Source: CAD feature listing. Evaluate the final solid. Frame: model axes, mm. Face numbers are marked on the shaded views. Round coordinates to 2 decimals unless told otherwise and drop trailing zeros. Write each loop counter-clockwise with the first axis right and the second up, starting at its lowest first coordinate (ties: lowest second). Pieces come first, ordered by that corner, then holes.
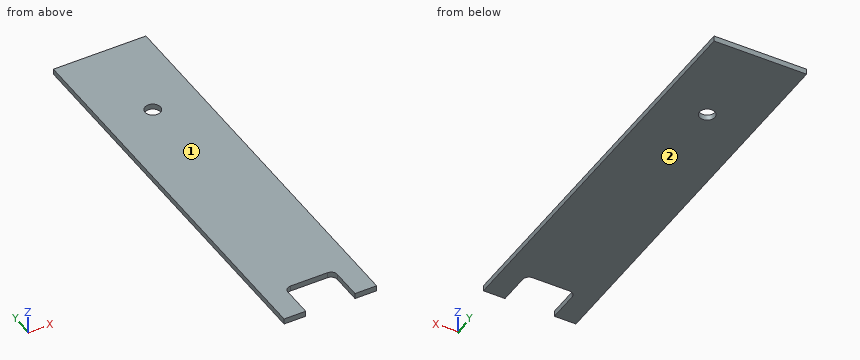
```python
from build123d import *

# Parameters (mm, degrees)
ESBO_O1_W                = 30
ESBO_O1_H                = 130
RESSALTO_EXTRUS_O1_DEPTH = 1.8
ESBO_O2_R                = 2.5
CORTE_EXTRUS_O1_DEPTH    = 10
CORTE_EXTRUS_O2_DEPTH    = 10.2


with BuildPart() as part:
    # Esboço1 → Ressalto-extrusão1 (new body)
    with BuildSketch(Plane.XY):
        with Locations((-11.632173448, -41.380470016)):
            Rectangle(ESBO_O1_W, ESBO_O1_H)
    extrude(amount=RESSALTO_EXTRUS_O1_DEPTH)

    # Esboço2 → Corte-extrusão1 (cut)
    with BuildSketch(Plane(origin=(0, 0, 0), x_dir=(-1, 0, 0), z_dir=(0, 0, -1))):
        with Locations((11.517661918, -6.126398996)):
            Circle(ESBO_O2_R)
    extrude(amount=-CORTE_EXTRUS_O1_DEPTH, mode=Mode.SUBTRACT)

    # Esboço3 → Corte-extrusão2 (cut)
    with BuildSketch(Plane(origin=(0, 0, 0), x_dir=(-1, 0, 0), z_dir=(0, 0, -1))):
        with BuildLine():
            Line((3.632173448, -106.380470016), (19.632173448, -106.380470016))
            Line((19.632173448, -106.380470016), (19.632173448, -96.380470016))
            ThreePointArc((19.632173448, -96.380470016), (19.04638701, -94.966256454), (17.632173448, -94.380470016))
            Line((17.632173448, -94.380470016), (5.632173448, -94.380470016))
            ThreePointArc((5.632173448, -94.380470016), (4.217959885, -94.966256454), (3.632173448, -96.380470016))
            Line((3.632173448, -96.380470016), (3.632173448, -106.380470016))
        make_face()
    extrude(amount=-CORTE_EXTRUS_O2_DEPTH, mode=Mode.SUBTRACT)


solid = part.part
```
Q1. Pin query (flat end, axial travel): P1, Ø0.5, axis at x = -9.5, z = 1, coming from the -Y side. Return the tip coordinate at first contact, or that it passes through.
Q2. Mould query, pull axis Z, two halves, no side actions, for the marked faces 1 and 2. Classes: pulls with the +Z half, pulls with the -Z half, needs draft (parallel to the pull), parting line crosses it, or undercut.
Q3. Section query A-A, the plane x = -11. Output: boundary loops of the cut face in (y, z), and give its area (3 significant figures).
Q4. Line query: line 1 (Y direction, x = -5.75, z = 1.1); line 2 (Y direction, x = -13.5, z = 0.6); line 3 (Y direction, x = -9.5, z = 1.15). Output: solid intervals per line, ascending.
Q5. Section query B-B, the plane z = 0.3. Output: boundary loops of the cut face in (x, y), and give its area (3 significant figures).
Filled in:
1. P1: stops at y = -94.38
2. face 1: pulls with the +Z half
2. face 2: pulls with the -Z half
3. outline: (-94.38, 0) - (-8.57, 0) - (-8.57, 1.8) - (-94.38, 1.8) - close; (-3.68, 0) - (23.62, 0) - (23.62, 1.8) - (-3.68, 1.8) - close
3. area: 204 mm2
4. line 1: y = -94.38 to 23.62
4. line 2: y = -94.38 to -7.65, -4.6 to 23.62
4. line 3: y = -94.38 to -7.6, -4.65 to 23.62
5. outline: (-26.63, -106.38) - (-19.63, -106.38) - (-19.63, -96.38) arc R2 cw to (-17.63, -94.38) - (-5.63, -94.38) arc R2 cw to (-3.63, -96.38) - (-3.63, -106.38) - (3.37, -106.38) - (3.37, 23.62) - (-26.63, 23.62) - close; hole circle Ø5 at (-11.52, -6.13)
5. area: 3,690 mm2
